Design review of the part built by this model. Coordinates are the model's own, in mm. A direction names the side the tool comes from. Coordinates: 2 decimals unless noted, no trailing zeros. Loops run counter-clockwise (first coordinate to the right, second up) from the corner with the lowest first, then second, coordinate; pieces in that order, holes last. Notation, with made-up numbers: (73.25, -18) -> (116.25, -18) arc R26 ccw to (116.25, 13) -> close; hole circle Ø2 at (-18, -39). An arc over 180 degrees is marked (long way). Answer as a JSON object with one key per item and string values.
Autodesk Inventor part; units mm, degrees
ref_plane "Work Plane3" through (0, 20, -40.5) normal (0, 0, -1) x (-1, 0, 0)
ref_plane "Work Plane4" through (-15, 20, -25.9808) normal (-0.5, 0, -0.866) x (0, -1, 0)
ref_plane "YZ Plane" through (0, 0, 0) normal (1, 0, 0) x (0, 1, 0)
sketch "Sketch1" plane through (0, 0, 0) normal (0, 1, 0) x (-1, 0, 0)
  circle A0 centre (0, 0) radius 30
  circle A1 centre (0, 0) radius 27.5
  circle A2 centre (0, -37) radius 3.5
  arc A3 (13.2962, -26.8926) -> (3.3005, -38.1648) centre (22.1604, -44.8209) ccw
  line L0 (0, -39.6745) -> (0, -15.9391) construction
  arc A4 (-3.3005, -38.1648) -> (-13.2962, -26.8926) centre (-22.1604, -44.8209) ccw
  line L1 (47.8103, 0) -> (-62.0389, 0) construction
  circle A5 centre (0, -37) radius 2
  circle A6 centre (32.0429, -18.5) radius 3.5
  circle A7 centre (32.0429, -18.5) radius 2
  arc A8 (31.4015, -21.9407) -> (16.6415, -24.9612) centre (27.7359, -41.6019) ccw
  arc A9 (29.9378, -1.9314) -> (34.7019, -16.2241) centre (49.8963, -3.219) ccw
  circle A10 centre (32.0429, 18.5) radius 3.5
  circle A11 centre (32.0429, 18.5) radius 2
  arc A12 (34.7019, 16.2241) -> (29.9378, 1.9314) centre (49.8963, 3.219) ccw
  arc A13 (16.6415, 24.9612) -> (31.4015, 21.9407) centre (27.7359, 41.6019) ccw
  circle A14 centre (0, 37) radius 3.5
  circle A15 centre (0, 37) radius 2
  arc A16 (3.3005, 38.1648) -> (13.2962, 26.8926) centre (22.1604, 44.8209) ccw
  arc A17 (-13.2962, 26.8926) -> (-3.3005, 38.1648) centre (-22.1604, 44.8209) ccw
  circle A18 centre (-32.0429, 18.5) radius 3.5
  circle A19 centre (-32.0429, 18.5) radius 2
  arc A20 (-31.4015, 21.9407) -> (-16.6415, 24.9612) centre (-27.7359, 41.6019) ccw
  arc A21 (-29.9378, 1.9314) -> (-34.7019, 16.2241) centre (-49.8963, 3.219) ccw
  circle A22 centre (-32.0429, -18.5) radius 3.5
  circle A23 centre (-32.0429, -18.5) radius 2
  arc A24 (-34.7019, -16.2241) -> (-29.9378, -1.9314) centre (-49.8963, -3.219) ccw
  arc A25 (-16.6415, -24.9612) -> (-31.4015, -21.9407) centre (-27.7359, -41.6019) ccw
  point P0 (29.9378, 1.9314)
  point P1 (34.7019, 16.2241)
  point P2 (16.6415, 24.9612)
  point P3 (13.2962, 26.8926)
  point P4 (3.3005, 38.1648)
  point P5 (-13.2962, 26.8926)
  point P6 (-16.6415, 24.9612)
  point P7 (-31.4015, 21.9407)
  point P8 (-29.9378, 1.9314)
  point P9 (-29.9378, -1.9314)
  point P10 (-16.6415, -24.9612)
  point P11 (-3.3005, -38.1648)
  point P12 (16.6415, -24.9612)
  point P13 (31.4015, -21.9407)
  point P14 (29.9378, -1.9314)
  dimension "d16" = 60
  dimension "d18" = 7
  dimension "d17" = 55
  dimension "d19" = 37
  dimension "d21" = 20
  dimension "d22" = 4
  dimension "d25" = 360
extrude "Extrusion5" add sketch "Sketch1" along normal blind 20
extrude "Extrusion6" add sketch "Sketch1" along normal blind 5 contours A1
sketch "Sketch4" plane through (0, 5, 0) normal (0, 1, 0) x (1, 0, 0)
  circle A0 centre (0, 0) radius 27.5
ref_plane "Work Plane3" through (0, 20, -40.5) normal (0, 0, -1) x (-1, 0, 0)
sketch "Sketch5" plane through (0, 20, -40.5) normal (0, 0, -1) x (-1, 0, 0)
  line L0 (-13.2962, -20) -> (-16.6415, -20)
  line L1 (-13.2962, 0) -> (-16.6415, 0)
  circle A0 centre (-15, -8) radius 5
  circle A1 centre (-15, -8) radius 3
  line L2 (3.3005, -20) -> (-3.3005, -20)
  circle A2 centre (20.2025, -6) radius 1.5
  point P0 (0, -20)
  point P1 (0, -20)
  dimension "d33" = 10
  dimension "d34" = 6
  dimension "d35" = 8
  dimension "d36" = 15
  dimension "d41" = 3
extrude "Extrusion7" add sketch "Sketch5" against normal up to surface contours A0
extrude "Extrusion8" cut sketch "Sketch5" against normal up to surface contours A1
ref_plane "Work Plane4" through (-15, 20, -25.9808) normal (-0.5, 0, -0.866) x (0, -1, 0)
sketch "Sketch6" plane through (-15, 20, -25.9808) normal (-0.5, 0, -0.866) x (0, -1, 0)
  circle A0 centre (12, 0) radius 1.5
  line L0 (20, 1.9314) -> (20, -1.9314)
  point P0 (20, 0)
  point P1 (20, 0)
  point P2 (20, 0)
  dimension "d42" = 3
  dimension "d43" = 8
extrude "Extrusion9" cut sketch "Sketch6" against normal up to surface
sketch "Sketch8" plane through (0, 5, 0) normal (0, 1, 0) x (1, 0, 0)
  circle A0 centre (0, 0) radius 27.5
  circle A1 centre (0, 4) radius 4
  circle A2 centre (0, 4) radius 22.5
  dimension "d57" = 8
  dimension "d58" = 45
  dimension "d59" = 4
extrude "Extrusion11" add sketch "Sketch8" along normal blind 5 contours A1
properties part number "carcaza motor"
1) Add section C-C, the plane y = 2.75. Count the separate pieces of the cut face and the enclosed holes in it, and give its area (3 significant figures).
Completed:
{"separate pieces": "1", "enclosed holes": "6", "area": "3,430 mm²"}
2) Add section B-B, the plane x = -1. Give the boundary of the cut face in (y, z).
Completed:
{"outline": "(0, -40.35) -> (20, -40.35) -> (20, -38.73) -> (0, -38.73) -> close; (0, -35.27) -> (20, -35.27) -> (20, -27.48) -> (5, -27.48) -> (5, -7.87) -> (10, -7.87) -> (10, -0.13) -> (5, -0.13) -> (5, 27.48) -> (20, 27.48) -> (20, 35.27) -> (0, 35.27) -> close; (0, 38.73) -> (20, 38.73) -> (20, 40.35) -> (0, 40.35) -> close"}
3) The part is to be moulded in two halves that separate along Z. For faces 1 (the cylindrical face through (14.98, 18.33, -25.99)), 2 (the cylindrical face through (34.04, 9.86, -18.59)), 3 (the flat face through (5.4, 20, 27.2)), say which applies: pulls with the +Z half, pulls with the -Z half, needs draft (parallel to the pull), parting line crosses it, or undercut.
Completed:
{"face 1": "pulls with the -Z half", "face 2": "undercut", "face 3": "needs draft"}
4) Clearance check with flat-ended pins moving along their axes: pin 1 Ø2.5 at (x, z) = (1, -4) entering from +Y; pin 2 Ø2 at (y, z) = (14, -14) entering from +X; pin 3 Ø1 at (y, z) = (18, -8.5) entering from +X. State where each tip first meets the part, or that it passes through.
Completed:
{"pin 1": "y = 10", "pin 2": "x = 33.73", "pin 3": "x = 30.75"}
5) For faces 4 (the cylindrical face through (30.96, 9.86, 9.65)), 5 (the cylindrical face through (18, 12, -31)), 6 (the cylindrical face through (5.961, 12.395, 26.846)), list the 3-axis set-ups (+Z, -Z, +X, -X, +Y, -Y) from which the entire face can be reached by the end or side of a thin tool; tool diameter is ignored.
Completed:
{"face 4": "+X, +Y, -Y", "face 5": "-Z", "face 6": "+Y"}
6) Add section D-D, the plane z = 18.5. Give the boundary of the cut face in (x, y), and give its area (3 significant figures).
Completed:
{"outline": "(-35.54, 0) -> (-34.04, 0) -> (-34.04, 20) -> (-35.54, 20) -> close; (-30.04, 0) -> (30.04, 0) -> (30.04, 20) -> (20.35, 20) -> (20.35, 5) -> (-20.35, 5) -> (-20.35, 20) -> (-30.04, 20) -> close; (34.04, 0) -> (35.54, 0) -> (35.54, 20) -> (34.04, 20) -> close", "area": "651 mm²"}
7) Add section A-A, the plane z = -37. Give the boundary of the cut face in (x, y), and give its area (3 significant figures).
Completed:
{"outline": "(-3.75, 0) -> (-2, 0) -> (-2, 20) -> (-3.75, 20) -> close; (2, 0) -> (3.75, 0) -> (3.75, 20) -> (2, 20) -> close; circle Ø10 at (15, 12); hole circle Ø6 at (15, 12)", "area": "120 mm²"}
8) Wall thickness on probe 1 along Z at (x, y) = (0, 7.5); probe 2 along Z at (x, y) = (0, 16); probe 3 along Y at (x, z) = (21.5, -4.5): over which ranges is each line inside the solid? List them lowest first.
Completed:
{"probe 1": "-40.5 to -39, -35 to -27.5, -8 to 0, 27.5 to 35, 39 to 40.5", "probe 2": "-40.5 to -39, -35 to -27.5, 27.5 to 35, 39 to 40.5", "probe 3": "0 to 5"}
